from build123d import *

# Parameters (mm, degrees)
F0_R     = 12.5
F1_DEPTH = 50
F2_R     = 5
F3_DEPTH = 29.8360184767


with BuildPart() as f1:
    # F0 (on Front) → F1 (new body)
    with BuildSketch(Plane.XZ):
        Polygon((46.8509476544, 20.2477943437), (-4.7790577234, 50.8148116121), (-49.8045677617, 11.1574863645), (-26.0018579483, -43.9191058098), (33.7345357789, -38.3009865105), align=None)
        Circle(F0_R, mode=Mode.SUBTRACT)
    extrude(amount=F1_DEPTH)

    # F2 (on face) → F3 (cut, through all)
    with BuildSketch(Plane(origin=(21.0359449655, 0, 35.5313029779), x_dir=(0.8605000896, 0, -0.5094502878), z_dir=(0.5094502878, 0, 0.8605000896))):
        with Locations((0, -25)):
            Circle(F2_R)
    extrude(amount=-F3_DEPTH, mode=Mode.SUBTRACT)


solid = f1.part
CAD build for the part. Positions are in the model's coordinates, mm. Give positions to 0.01 mm unless a question says otherwise; leave off trailing zeros. Write each loop counter-clockwise with the first axis right and the second up, starting at its lowest first coordinate (ties: lowest second). Pieces come first, ordered by that corner, then holes. Notation, with made-up numbers: (-21.75, 86.5) - (-8.75, 86.5) arc R23 cw to (-8.75, 94.5) - close; hole circle Ø6 at (9, 49). An arc over 180 degrees is marked (long way). Put each result on its own line as item: value.
(1) Saw through at D-D (x = -43). List the corners of the cut face in (y, z), then the cut area to 3 significant figures.
Working result:
outline: (-50, -4.59) - (0, -4.59) - (0, 17.15) - (-50, 17.15) - close
area: 1,090 mm^2
(2) Saw through at C-C (x = 0). List the corners of the cut face in (y, z).
Working result:
outline: (-50, -41.47) - (0, -41.47) - (0, -12.5) - (-50, -12.5) - close; (-50, 12.5) - (0, 12.5) - (0, 47.99) - (-50, 47.99) - close
(3) Saw through at B-B (z = 0). List the corners of the cut face in (x, y), then the cut area to 3 significant figures.
Working result:
outline: (-44.98, -50) - (-12.5, -50) - (-12.5, 0) - (-44.98, 0) - close; (12.5, -50) - (42.31, -50) - (42.31, 0) - (12.5, 0) - close
area: 3,110 mm^2
(4) Saw through at A-A (y = -45.5). List the corners of the cut face in (x, z).
Working result:
outline: (-49.8, 11.16) - (-26, -43.92) - (33.73, -38.3) - (46.85, 20.25) - (-4.78, 50.81) - close; hole circle Ø25 at (0, 0)
(5) Wall check: L1, parallel to Z at x = 0, y = -18.5; L2, parallel to X at y = -23.5, z = 7; L3, parallel to X at y = -46.5, z = -11. Give the ranges that are in metal, low to high.
Working result:
L1: -41.47 to -12.5, 12.5 to 47.99
L2: -48.01 to -10.36, 10.36 to 43.88
L3: -40.23 to -5.94, 5.94 to 39.85
(6) Drop flat-ended pins along their axis: pin 1 Ø10 at (y, z) = (-17.5, -23) entering from +X; pin 2 Ø12 at (x, y) = (-7.5, -29.5) entering from -Z; pin 3 Ø1 at (y, z) = (-34.5, 36) entering from -X. Give the stop position or say it passes through.
Working result:
pin 1: x = 38.28
pin 2: z = -42.74
pin 3: x = -22.17
(7) Pull direction Z, two halves, no side cores. Call faces 1 (the flat face through (-26.98, -24.65, 31.26)), 2 (the cylindrical face through (-9.92, -24.65, -7.606)), 3 (the flat face through (-38.07, -24.65, -15.995)), 4 (the cylindrical face through (12.61, -29.88, 23.43)): released by +Z, released by -Z, zero draft, split by the parting line, or undercut.
Working result:
face 1: released by +Z
face 2: undercut
face 3: released by -Z
face 4: undercut
